from build123d import *

# Parameters (mm, degrees)
SKETCH1_R           = 21.8
BOSS_EXTRUDE1_DEPTH = 21
CHAMFER1_SIZE       = 1
SKETCH2_R           = 2.1
CUT_EXTRUDE1_DEPTH  = 5.8


with BuildPart() as part:
    # Sketch1 → Boss-Extrude1 (new body)
    with BuildSketch(Plane.XY):
        with Locations(Location((0, 0, 0), (0, 0, 180))):
            Circle(SKETCH1_R)
    extrude(amount=BOSS_EXTRUDE1_DEPTH)

    # Chamfer1
    chamfer1_edges = [part.edges().sort_by_distance(p)[0] for p in [
        (21.8, 0, 0),
        (21.8, 0, 21),
    ]]
    chamfer(chamfer1_edges, length=CHAMFER1_SIZE)

    # Sketch2 → Cut-Extrude1 (cut)
    with BuildSketch(Plane.XY.offset(21)):
        Circle(SKETCH2_R)
    extrude(amount=-CUT_EXTRUDE1_DEPTH, mode=Mode.SUBTRACT)


solid = part.part
The model under review builds one solid part; all positions refer to its coordinate system, in mm. A direction names the side the tool comes from. Coordinates: 2 decimals unless noted, no trailing zeros. Loops run counter-clockwise (first coordinate to the right, second up) from the corner with the lowest first, then second, coordinate; pieces in that order, holes last. Notation, with made-up numbers: M -10.5,42.5 L -4.5,42.5 A19 cw -4.5,52.5 Z; hole C -3,60.5 d4. An arc over 180 degrees is marked long. Put each result on its own line as item: value. Start each with the question number.
Q1. For faces 1 (the flat face through (0, 0, 15.2)), 2 (the flat face through (0, 0, 0)), list the 3-axis set-ups (+Z, -Z, +X, -X, +Y, -Y) from which the entire face can be reached by the end or side of a thin tool; tool diameter is ignored.
Q2. Clearance check with flat-ended pins moving along their axes: pin 1 (10 mm diameter, centred on x = 8, z = 8, fed in from -Y); pin 2 (10 mm diameter, centred on x = -4, z = 4.5, fed in from -Y); pin 3 (1 mm diameter, centred on x = -5.5, z = 17.5, fed in from +Y); pin 4 (5.5 mm diameter, centred on x = 0, y = 0, fed in from -Z). State where each tip first meets the part, or that it passes through.
Q3. Wall thickness on line 1 (Y direction, x = 0, z = 19.3); line 2 (X direction, y = -0.5, z = 2.25); line 3 (Y direction, x = 12, z = 11.25): over which ranges is each line inside the solid? List them lowest first.
Q4. Add section A-A (x = 0). Write out the cut boundary in (y, z), and give its area (3 significant figures).
Q5. The part is to be moulded in two halves that separate along Y. For faces 3 (the cylindrical face through (2.003, 0.631, 18.141)), 4 (the cylindrical face through (-10.06, 19.34, 10.37)), 5 (the flat face through (0, 4, 21)), say which applies: +Y half, -Y half, draft (parallel to the pull), parting line (faces both ways), or undercut.
Q6. Add section C-C (z = 3). Write out the cut boundary in (x, y), and give its area (3 significant figures).
Answers:
1. face 1: +Z
1. face 2: -Z, +X, -X, +Y, -Y
2. pin 1: stops at y = -21.59
2. pin 2: stops at y = -21.8
2. pin 3: stops at y = 21.22
2. pin 4: stops at z = 0
3. line 1: y = -21.8 to -2.1, 2.1 to 21.8
3. line 2: x = -21.79 to 21.79
3. line 3: y = -18.2 to 18.2
4. outline: M -21.8,1 L -20.8,0 L 20.8,0 L 21.8,1 L 21.8,20 L 20.8,21 L 2.1,21 L 2.1,15.2 L -2.1,15.2 L -2.1,21 L -20.8,21 L -21.8,20 Z
4. area: 889 mm^2
5. face 3: undercut
5. face 4: parting line
5. face 5: draft
6. outline: C 0,0 d43.6
6. area: 1,490 mm^2
